Source: CAD feature listing. Evaluate the final solid. Frame: model axes, mm. Face numbers are marked on the shaded views. A direction names the side the tool comes from. Round coordinates to 2 decimals unless told otherwise and drop trailing zeros. Loops run counter-clockwise (first coordinate to the right, second up) from the corner with the lowest first, then second, coordinate; pieces in that order, holes last. Notation, with made-up numbers: M 7.5,17.5 L 25.5,17.5 A23 ccw 25.5,35.5 Z; hole C -14,29 d8. An arc over 180 degrees is marked long. Answer as CSV lines item,"result". Start each with the question number.
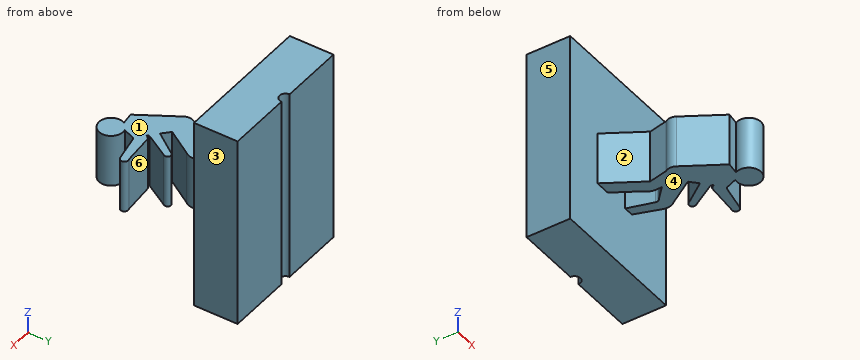
```python
from build123d import *

# Parameters (mm, degrees)
F0_W     = 80
F0_H     = 110
F1_DEPTH = 25
F3_DEPTH = 122.9
F5_DEPTH = 15


with BuildPart() as f1:
    # F0 (on Front) → F1 (new body)
    with BuildSketch(Plane.XZ):
        with Locations((-8.13742, 3.912851)):
            Rectangle(F0_W, F0_H)
    extrude(amount=F1_DEPTH)

    # F2 (on face) → F3 (cut)
    with BuildSketch(Plane(origin=(0, 0, -51.087149), x_dir=(1, 0, 0), z_dir=(0, 0, -1))):
        with BuildLine():
            ThreePointArc((-11.533121, 0), (-8.13742, -3.395701), (-4.741719, 0))
            Line((-4.741719, 0), (-11.533121, 0))
        make_face()
        with BuildLine():
            Line((-11.533121, 0), (-4.741719, 0))
            ThreePointArc((-4.741719, 0), (-8.13742, 3.395701), (-11.533121, 0))
        make_face()
    extrude(amount=-F3_DEPTH, mode=Mode.SUBTRACT)

    # F4 (on Top) → F5 (join, symmetric)
    with BuildSketch(Plane.XY):
        with BuildLine():
            Line((-25.619638, -24.679836), (-12.538977, -46.366195))
            Line((-12.538977, -46.366195), (-14.788412, -56.985627))
            ThreePointArc((-14.788412, -56.985627), (-15.806818, -59.965228), (-15.021523, -63.014571))
            Line((-15.021523, -63.014571), (-2.031637, -84.550433))
            Line((-2.031637, -84.550433), (4.691661, -83.66965))
            ThreePointArc((4.691661, -83.66965), (15.085472, -92.244671), (9.213005, -80.117164))
            Line((9.213005, -80.117164), (11.628102, -73.915706))
            Line((11.628102, -73.915706), (12.371922, -73.123584))
            Line((12.371922, -73.123584), (27.714186, -70.096895))
            ThreePointArc((27.714186, -70.096895), (29.362088, -67.253343), (26.327906, -65.990366))
            Line((26.327906, -65.990366), (8.524408, -67.434899))
            Line((8.524408, -67.434899), (7.119579, -68.6341))
            Line((7.119579, -68.6341), (6.93642, -69.498782))
            Line((6.93642, -69.498782), (6.318386, -69.050649))
            Line((6.318386, -69.050649), (6.318386, -67.899771))
            Line((6.318386, -67.899771), (14.191412, -54.533935))
            ThreePointArc((14.191412, -54.533935), (13.865423, -51.491249), (10.974195, -52.49375))
            Line((10.974195, -52.49375), (1.951577, -64.937122))
            Line((1.951577, -64.937122), (-2.338045, -60.909065))
            Line((-2.338045, -60.909065), (6.969567, -46.276149))
            ThreePointArc((6.969567, -46.276149), (8.484232, -43.032088), (8.229074, -39.460949))
            Line((8.229074, -39.460949), (3.24195, -24.679836))
            Line((3.24195, -24.679836), (-2.338045, -24.679836))
            Line((-2.338045, -24.679836), (1.951577, -39.460949))
            ThreePointArc((1.951577, -39.460949), (1.878572, -40.948809), (0.905328, -42.076573))
            Line((0.905328, -42.076573), (-5.799454, -48.446116))
            Line((-5.799454, -48.446116), (-5.799454, -44.733086))
            ThreePointArc((-5.799454, -44.733086), (-6.321583, -42.158323), (-7.805476, -39.990356))
            Line((-7.805476, -39.990356), (-17.040393, -24.679836))
            Line((-17.040393, -24.679836), (-25.619638, -24.679836))
        make_face()
    extrude(amount=F5_DEPTH, both=True)


solid = f1.part
```
1) Section A-A, the plane z = 22.5. Return loops of the section in (x, y), and give its area (3 significant figures).
2) Contact query for flat-ended pins moving along their axis: pin 1 Ø1.3 at (y, z) = (-68.5, 4) entering from +X; pin 2 Ø1.1 at (y, z) = (-46.5, 1) entering from +X; pin 3 Ø6 at (y, z) = (-28.5, 41) entering from +X; pin 4 Ø2 at (x, z) = (-22.5, -23) entering from -Y. Output: stop coordinate, or through.
3) Section B-B, the plane x = -43. Return loops of the section in (y, z), and give its area (3 significant figures).
4) Ray query, line 1 along Y through (x, z) = (-13.5, 21); line 2 along Y through (x, z) = (-9, -14). Return the intervals inside material, ascending.
5) Mould query, pull axis X, two halves, no side actions, for the marked faces 4, 5 and 6. Classes: pulls with the +X half, pulls with the -X half, needs draft (parallel to the pull), parting line crosses it, or undercut.
6) Section C-C, the plane y = -76. Return loops of the section in (x, z).
7) Access query for the marked faces 1, 2 and 3. Directions: +Z, -Z, +X, -X, +Y, -Y. A direction counts if a zero-diameter tool reaches every point of the face in a straight line with its end or side. Return the directions, or none.
8) Section D-D, the plane x = -21.5. Return loops of the section in (y, z), and give its area (3 significant figures).
Findings below:
1,outline,"M -48.14,-25 L 31.86,-25 L 31.86,0 L -4.74,0 A3.4 cw -11.53,0 L -48.14,0 Z"
1,area,"1,980 mm²"
2,pin 1,"x = 29.48"
2,pin 2,"x = 7.22"
2,pin 3,"through"
2,pin 4,"y = -25"
3,outline,"M -25,-51.09 L 0,-51.09 L 0,58.91 L -25,58.91 Z"
3,area,"2,750 mm²"
4,line 1,"-25 to 0"
4,line 2,"-73 to -38.01, -25 to -3.28"
5,face 4,"needs draft"
5,face 5,"pulls with the -X half"
5,face 6,"undercut"
6,outline,"M -7.19,-15 L 10.82,-15 L 10.82,15 L -7.19,15 Z"
7,face 1,"+Z, +X, -X, -Y"
7,face 2,"+Z, -Z, -X"
7,face 3,"+Z, -Z, +X, +Y, -Y"
8,outline,"M -31.51,-15 L -25,-15 L -25,-51.09 L 0,-51.09 L 0,58.91 L -25,58.91 L -25,15 L -31.51,15 Z"
8,area,"2,950 mm²"
